Geometry: final body of the model. Coordinates: model frame, mm. Give positions to 0.01 mm unless a question says otherwise; leave off trailing zeros. Order: outer loops, then holes, each group sorted by start corner. A loop starts at its lowest first (then second) coordinate and runs counter-clockwise, first axis right, second up. Notation, with made-up numbers: (47.25, 60.25) - (58.25, 60.25) arc R8 cw to (58.25, 72.25) - close; hole circle Ø2 at (-8.75, -29.5). An arc over 180 degrees is marked (long way). Write item = value, one per line. Start each with the question number.
from build123d import *

# Parameters (mm, degrees)
SKETCH_1_R          = 1.75
EXTRUDE_2_DEPTH     = 2.5
SKETCH_2_W          = 43.174936718
SKETCH_2_H          = 3.770638763
SKETCH_2_W_2        = 34.014564127
CUT_EXTRUDE_1_DEPTH = 3.5
SKETCH_3_R          = 1.75
CUT_EXTRUDE_2_DEPTH = 3.5


with BuildPart() as part:
    # 草图1 → 凸台-拉伸2 (new body)
    with BuildSketch(Plane.XY):
        with BuildLine():
            ThreePointArc((-1.307031792, 5.855908802), (-5.975846633, -0.537826197), (-0.240433737, -5.995180699))
            Line((-0.240433737, -5.995180699), (49.499096381, -7.98995979))
            ThreePointArc((49.499096381, -7.98995979), (49.730212736, -7.997088254), (49.961421407, -7.999940468))
            Line((49.961421407, -7.999940468), (49.999999816, -8.000059532))
            Line((49.999999816, -8.000059532), (211.973766557, -8.499959518))
            ThreePointArc((211.973766557, -8.499959518), (220.496722576, -0.236020072), (212.445662896, 8.4883087))
            Line((212.445662896, 8.4883087), (50.655386612, 16.982806911))
            ThreePointArc((50.655386612, 16.982806911), (50.327806045, 16.995700989), (50, 17))
            ThreePointArc((50, 17), (48.630260069, 16.924725853), (47.2770171, 16.699810004))
            Line((47.2770171, 16.699810004), (-1.307031792, 5.855908802))
        make_face()
        Circle(SKETCH_1_R, mode=Mode.SUBTRACT)
        with Locations((50, 0)):
            Circle(SKETCH_1_R, mode=Mode.SUBTRACT)
        with Locations((212, 0)):
            Circle(SKETCH_1_R, mode=Mode.SUBTRACT)
    extrude(amount=EXTRUDE_2_DEPTH)

    # 草图2 → 切除-拉伸1 (cut, through all)
    with BuildSketch(Plane.XY.offset(2.5)):
        with BuildLine():
            Line((59.758236221, 8.91451918), (74.115618559, 8.91451918))
            ThreePointArc((74.115618559, 8.91451918), (77.403568713, 5.626569026), (74.115618559, 2.338618872))
            Line((74.115618559, 2.338618872), (59.758236221, 2.338618872))
            ThreePointArc((59.758236221, 2.338618872), (56.470286067, 5.626569026), (59.758236221, 8.91451918))
        make_face()
        with Locations((111.440293999, 3.490211277)):
            Rectangle(SKETCH_2_W, SKETCH_2_H)
        with Locations((165.07921871, 3.490211277)):
            Rectangle(SKETCH_2_W_2, SKETCH_2_H)
    extrude(amount=-CUT_EXTRUDE_1_DEPTH, mode=Mode.SUBTRACT)

    # 草图3 → 切除-拉伸2 (cut, through all)
    with BuildSketch(Plane.XY.offset(2.5)):
        with BuildLine():
            ThreePointArc((84.93827664, 3.287023225), (83.18827664, 5.037023225), (81.43827664, 3.287023225))
            Line((81.43827664, 3.287023225), (84.93827664, 3.287023225))
        make_face()
        with BuildLine():
            Line((84.93827664, 3.287023225), (81.43827664, 3.287023225))
            ThreePointArc((81.43827664, 3.287023225), (83.18827664, 1.537023225), (84.93827664, 3.287023225))
        make_face()
        with Locations((193.595777353, 3.287023225)):
            Circle(SKETCH_3_R)
    extrude(amount=-CUT_EXTRUDE_2_DEPTH, mode=Mode.SUBTRACT)


solid = part.part
Q1. Section B-B, the plane z = 1.55. Count the separate pieces of the cut face and the enclosed holes in it, then the cut area to 3 significant figures.
Q2. Section C-C, the plane y = 14.25. Return the cut outline in (x, z).
Q3. Material intervals for line 1 along Y through (x, z) = (50, 0.5); line 2 along Y through (x, z) = (212, 1.9); line 3 along X through (y, z) = (-0.5, 1.5), sorted ascending. Write a range as from..to.
Q4. Pull-direction query (Y, two-part tool) for faces 1 (the cylindrical face through (84.937, 3.21, 1.268)), 2 (the flat face through (106, -1, 2.5)), 3 (the cylindrical face through (-6, 0, 1)); classes: +Y half, -Y half, draft (parallel to the pull), parting line (faces both ways), or undercut.
Q5. Section A-A, the plane x = 157.5. Return the cut outline in (y, z), then the cut area to 3 significant figures.
Q6. Contact query for flat-ended pins moving along their axis: pin 1 (2 mm diameter, centred on x = 193.6, y = 3.29, fed in from -Z); pin 2 (0.8 mm diameter, centred on x = 68.5, z = 1, fed in from -Y); pin 3 (1.2 mm diameter, centred on y = 3.5, z = 0.5, fed in from -X); pin 4 (1.2 mm diameter, centred on x = 66.5, z = 2, fed in from +Y). Output: stop coordinate, or through.
The answers:
q1.separate_pieces = 1
q1.enclosed_holes = 8
q1.area = 4,040 mm²
q2.outline = (36.3, 0) - (102.71, 0) - (102.71, 2.5) - (36.3, 2.5) - close
q3.line_1 = -8..-1.75, 1.75..17
q3.line_2 = -8.5..-1.75, 1.75..8.51
q3.line_3 = -5.98..-1.68, 1.68..48.32, 51.68..210.32, 213.68..220.49
q4.face_1 = undercut
q4.face_2 = draft
q4.face_3 = parting line
q5.outline = (-8.33, 0) - (1.6, 0) - (1.6, 2.5) - (-8.33, 2.5) - close; (5.38, 0) - (11.37, 0) - (11.37, 2.5) - (5.38, 2.5) - close
q5.area = 39.8 mm²
q6.pin_1 = through
q6.pin_2 = -8.06
q6.pin_3 = -5.25
q6.pin_4 = 16.18
